Input: part model. Units: mm. Frame: model coordinates. A direction names the side the tool comes from. Give positions to 0.01 mm unless a question says otherwise; leave off trailing zeros. Order: outer loops, then holes, each group sorted by start corner. A loop starts at its lowest first (then second) coordinate and runs counter-clockwise, first axis right, second up. Notation, with made-up numbers: (-19, 51.25) - (32, 51.25) arc R20 ccw to (32, 77.25) - close; hole circle Ø10 at (18.5, 10). An arc over 180 degrees is marked (long way). Use a Markdown table: item, result.
from build123d import *

# Parameters (mm, degrees)
SKETCH1_R           = 4.5
BOSS_EXTRUDE1_DEPTH = 150
SKETCH2_R           = 2
SKETCH2_R_2         = 11.05
CUT_EXTRUDE1_DEPTH  = 162.692656416
SKETCH3_R           = 2.5
CUT_EXTRUDE2_DEPTH  = 162.692656416


with BuildPart() as part:
    # Sketch1 → Boss-Extrude1 (new body)
    with BuildSketch(Plane.XY):
        with BuildLine():
            Line((-2.5, 59.16515139), (-2.5, 9.16515139))
            ThreePointArc((-2.5, 9.16515139), (0, -9.5), (2.5, 9.16515139))
            Line((2.5, 9.16515139), (2.5, 59.16515139))
            Line((2.5, 59.16515139), (-2.5, 59.16515139))
        make_face()
        Circle(SKETCH1_R, mode=Mode.SUBTRACT)
    extrude(amount=BOSS_EXTRUDE1_DEPTH)

    # Sketch2 → Cut-Extrude1 (cut, through all)
    with BuildSketch(Plane.ZY.offset(2.5)):
        with Locations(Location((9.5, 50.5, 0), (0, 0, 270))):
            Circle(SKETCH2_R)
        with Locations(Location((40.5, 50.5, 0), (0, 0, 270))):
            Circle(SKETCH2_R)
        with Locations(Location((40.5, 19.5, 0), (0, 0, 270))):
            Circle(SKETCH2_R)
        with Locations(Location((9.5, 19.5, 0), (0, 0, 270))):
            Circle(SKETCH2_R)
        with Locations(Location((25, 35, 0), (0, 0, 270))):
            Circle(SKETCH2_R_2)
    extrude(amount=-CUT_EXTRUDE1_DEPTH, mode=Mode.SUBTRACT)

    # Sketch3 → Cut-Extrude2 (cut, through all)
    with BuildSketch(Plane.ZY.offset(2.5)):
        with Locations(Location((113.5, 35, 0), (0, 0, 270))):
            Circle(SKETCH3_R)
        with Locations(Location((136.5, 35, 0), (0, 0, 270))):
            Circle(SKETCH3_R)
    extrude(amount=-CUT_EXTRUDE2_DEPTH, mode=Mode.SUBTRACT)


solid = part.part
1. Pin query (flat end, axial travel): pin 1 (5 mm diameter, centred on y = 50.5, z = 40.5, fed in from +X); pin 2 (4 mm diameter, centred on x = -5, z = 31, fed in from +Y); pin 3 (2 mm diameter, centred on y = 15.5, z = 43.5, fed in from -X). Return the tip coordinate at first contact, or that it passes through.
Response:
| item | result |
|---|---|
| pin 1 | stops at x = 2.5 |
| pin 2 | stops at y = 9.01 |
| pin 3 | stops at x = -2.5 |
2. Section query B-B (y = 19.5). Return loops of the section in (x, z), then the cut area to 3 significant figures.
Response:
| item | result |
|---|---|
| outline | (-2.5, 0) - (2.5, 0) - (2.5, 7.5) - (-2.5, 7.5) - close; (-2.5, 11.5) - (2.5, 11.5) - (2.5, 38.5) - (-2.5, 38.5) - close; (-2.5, 42.5) - (2.5, 42.5) - (2.5, 150) - (-2.5, 150) - close |
| area | 710 mm^2 |
3. Material intervals for line 1 along Z through (x, y) = (-0.05, 50.5); line 2 along Y through (x, z) = (-1.4, 136.5); line 3 along Z through (x, y) = (-0.25, 35), sorted ascending.
Response:
| item | result |
|---|---|
| line 1 | z = 0 to 7.5, 11.5 to 38.5, 42.5 to 150 |
| line 2 | y = -9.4 to -4.28, 4.28 to 32.5, 37.5 to 59.17 |
| line 3 | z = 0 to 13.95, 36.05 to 111, 116 to 134, 139 to 150 |
4. Set-up query: faces 4 (the face through (-0.035, 19.76, 11.483)), 5 (the face through (-2.5, 35, 74)). Return all of +Z, -Z, +X, -X, +Y, -Y with unobstructed straight access to the full face (end or side cutting, diameter ignored); none if empty.
Response:
| item | result |
|---|---|
| face 4 | +X, -X |
| face 5 | +Z, -Z, -X, +Y |
5. Section query A-A (z = 113.5). Return loops of the section in (x, y), then the cut area to 3 significant figures.
Response:
| item | result |
|---|---|
| outline | (-2.5, 9.17) arc R9.5 ccw (long way) to (2.5, 9.17) - (2.5, 32.5) - (-2.5, 32.5) - close; (-2.5, 37.5) - (2.5, 37.5) - (2.5, 59.17) - (-2.5, 59.17) - close; hole circle Ø9 at (0, 0) |
| area | 444 mm^2 |
6. Section query D-D (z = 9.5). Return loops of the section in (x, y).
Response:
| item | result |
|---|---|
| outline | (-2.5, 9.17) arc R9.5 ccw (long way) to (2.5, 9.17) - (2.5, 17.5) - (-2.5, 17.5) - close; (-2.5, 21.5) - (2.5, 21.5) - (2.5, 48.5) - (-2.5, 48.5) - close; (-2.5, 52.5) - (2.5, 52.5) - (2.5, 59.17) - (-2.5, 59.17) - close; hole circle Ø9 at (0, 0) |
7. Mould query, pull axis X, two halves, no side actions, for faces 1 (the face through (2.5, 34, 74)), 2 (the face through (-0.04, 33.66, 138.61)), 3 (the face through (-0.59, 4.46, 73.95)). Classes: pulls with the +X half, pulls with the -X half, needs draft (parallel to the pull), parting line crosses it, or undercut.
Response:
| item | result |
|---|---|
| face 1 | pulls with the +X half |
| face 2 | needs draft |
| face 3 | undercut |
8. Section query C-C (x = 0). State how many separate pieces and enclosed holes the cut face has, then the cut area to 3 significant figures.
Response:
| item | result |
|---|---|
| separate pieces | 2 |
| enclosed holes | 7 |
| area | 8,480 mm^2 |
